CAD build for the part. Positions are in the model's coordinates, mm. A direction names the side the tool comes from. Coordinates: 2 decimals unless noted, no trailing zeros. Order: outer loops, then holes, each group sorted by start corner. A loop starts at its lowest first (then second) coordinate and runs counter-clockwise, first axis right, second up. Notation, with made-up numbers: (20.25, 67.5) - (29.25, 67.5) arc R24 cw to (29.25, 80.5) - close; hole circle Ø7 at (43, 60.25). An arc over 180 degrees is marked (long way). Return JSON: item names as keys, results as strings.
from build123d import *

# Parameters (mm, degrees)
SKETCH1_R           = 5
BOSS_EXTRUDE1_DEPTH = 6
SKETCH2_R           = 13
CUT_EXTRUDE1_DEPTH  = 3
CUT_EXTRUDE1_DRAFT  = -30
SKETCH3_R           = 18
BOSS_EXTRUDE2_DEPTH = 48
SKETCH4_R           = 38
BOSS_EXTRUDE3_DEPTH = 10
SKETCH5_R           = 11.267949192
CUT_EXTRUDE2_DEPTH  = 25
SKETCH6_R           = 10
CUT_EXTRUDE3_DEPTH  = 76.55130707
SKETCH7_R           = 4
CUT_EXTRUDE4_DEPTH  = 87.856203002
FILLET1_R           = 2


with BuildPart() as part:
    # Sketch1 → Boss-Extrude1 (new, symmetric)
    with BuildSketch(Plane.XY):
        with BuildLine():
            Line((23.491540883, -8.552631579), (11.275939624, -42.105263158))
            ThreePointArc((11.275939624, -42.105263158), (0, -50), (-11.275939624, -42.105263158))
            Line((-11.275939624, -42.105263158), (-23.491540883, -8.552631579))
            ThreePointArc((-23.491540883, -8.552631579), (-25, 0), (-23.491540883, 8.552631579))
            Line((-23.491540883, 8.552631579), (-11.275939624, 42.105263158))
            ThreePointArc((-11.275939624, 42.105263158), (0, 50), (11.275939624, 42.105263158))
            Line((11.275939624, 42.105263158), (23.491540883, 8.552631579))
            ThreePointArc((23.491540883, 8.552631579), (25, 0), (23.491540883, -8.552631579))
        make_face()
        with Locations((0, -38)):
            Circle(SKETCH1_R, mode=Mode.SUBTRACT)
        with Locations((0, 38)):
            Circle(SKETCH1_R, mode=Mode.SUBTRACT)
    extrude(amount=BOSS_EXTRUDE1_DEPTH, both=True)


with BuildPart() as cut_extrude1_tool:
    # Sketch2 → Cut-Extrude1 (with draft: the straight prism first)
    with BuildSketch(Plane.XY.offset(6)):
        Circle(SKETCH2_R)
    extrude(amount=-CUT_EXTRUDE1_DEPTH)
    # Cut-Extrude1: the draft: its side faces are tilted about the plane it starts from
    cut_extrude1_sides = [cut_extrude1_tool.faces().sort_by_distance(p)[0] for p in [
        (-13, 0, 4.5),
    ]]
    draft(cut_extrude1_sides, Plane.XY.offset(6), CUT_EXTRUDE1_DRAFT)


with BuildPart() as part_1:
    add(part.part)

    # Cut-Extrude1: cut by cut_extrude1_tool
    add(cut_extrude1_tool.part, mode=Mode.SUBTRACT)

    # Sketch3 → Boss-Extrude2 (add)
    with BuildSketch(Plane(origin=(0, 0, -6), x_dir=(-1, 0, 0), z_dir=(0, 0, -1))):
        with Locations(Location((0, 0, 0), (0, 0, 180))):
            Circle(SKETCH3_R)
    extrude(amount=BOSS_EXTRUDE2_DEPTH)

    # Sketch4 → Boss-Extrude3 (add)
    with BuildSketch(Plane(origin=(0, 0, -54), x_dir=(-1, 0, 0), z_dir=(0, 0, -1))):
        Circle(SKETCH4_R)
    extrude(amount=BOSS_EXTRUDE3_DEPTH)

    # Sketch5 → Cut-Extrude2 (cut)
    with BuildSketch(Plane.XY.offset(3)):
        Circle(SKETCH5_R)
    extrude(amount=-CUT_EXTRUDE2_DEPTH, mode=Mode.SUBTRACT)

    # Sketch6 → Cut-Extrude3 (cut, through all)
    with BuildSketch(Plane.XY.offset(-22)):
        Circle(SKETCH6_R)
    extrude(amount=-CUT_EXTRUDE3_DEPTH, mode=Mode.SUBTRACT)

    # Sketch7 → Cut-Extrude4 (cut, through all)
    with BuildSketch(Plane.XY.offset(-54)):
        with Locations((0, 29)):
            Circle(SKETCH7_R)
        with Locations((25.11473671, 14.5)):
            Circle(SKETCH7_R)
        with Locations((25.11473671, -14.5)):
            Circle(SKETCH7_R)
        with Locations((0, -29)):
            Circle(SKETCH7_R)
        with Locations((-25.11473671, -14.5)):
            Circle(SKETCH7_R)
        with Locations((-25.11473671, 14.5)):
            Circle(SKETCH7_R)
    extrude(amount=-CUT_EXTRUDE4_DEPTH, mode=Mode.SUBTRACT)

    # Fillet1
    fillet1_edges = [part_1.edges().sort_by_distance(p)[0] for p in [
        (-18, 0, -54),
        (38, 0, -54),
    ]]
    fillet(fillet1_edges, radius=FILLET1_R)


solid = part_1.part
Item 1: Drop flat-ended pins along their axis: P1, Ø6, axis at x = 16, z = -18.5, coming from the -Y side; P2, Ø12, axis at y = -3, z = -34.5, coming from the -X side; P3, Ø12, axis at x = -2, z = -31.5, coming from the +Y side. Give the stop position or say it passes through.
Findings below:
{"P1": "stops at y = -12.45", "P2": "stops at x = -18", "P3": "stops at y = 18"}
Item 2: Band-saw the part on C-C, the plane z = -48. List the corners of the cut face in (x, y), then the cut area to 3 significant figures.
Findings below:
{"outline": "circle Ø36 at (0, 0); hole circle Ø20 at (0, 0)", "area": "704 mm²"}
Item 3: Band-saw the part on A-A, the plane z = 0. List the corners of the cut face in (x, y), then the cut area to 3 significant figures.
Findings below:
{"outline": "(-23.49, -8.55) - (-11.28, -42.11) arc R12 ccw to (11.28, -42.11) - (23.49, -8.55) arc R25 ccw to (23.49, 8.55) - (11.28, 42.11) arc R12 ccw to (-11.28, 42.11) - (-23.49, 8.55) arc R25 ccw to start; hole circle Ø22.54 at (0, 0); hole circle Ø10 at (0, -38); hole circle Ø10 at (0, 38)", "area": "2,870 mm²"}
Item 4: Band-saw the part on B-B, the plane x = 0. Count the separate pieces of the cut face and the enclosed holes in it, then the cut area to 3 significant figures.
Findings below:
{"separate pieces": "6", "enclosed holes": "0", "area": "1,810 mm²"}
Item 5: Wall check: L1, parallel to Y at x = 0, z = -61.5; L2, parallel to X at y = 14, z = -58; L3, parallel to Z at x = 5.5, y = 38.5. Give the ranges that are in metal, low to high. Write a range as [from, to].
Findings below:
{"L1": "y = [-38, -33], [-25, -10], [10, 25], [33, 38]", "L2": "x = [-35.33, -29.08], [-21.15, 21.15], [29.08, 35.33]", "L3": "z = [-6, 6]"}
Item 6: Mould opens along X. For faces 4 (the cylindrical face through (28.81, -16.03, -58.93)), 5 (the cylindrical face through (-25, 0, 0)), 6 (the cylindrical face through (0, 50, 0)) say: released by +X, released by -X, zero draft, split by the parting line, or undercut.
Findings below:
{"face 4": "undercut", "face 5": "released by -X", "face 6": "split by the parting line"}
Item 7: Which spindle directions (+Z, -Z, +X, -X, +Y, -Y) get a long thin tool onto all of the face, cutting with end or side? Do faces 1 (the cylindrical face through (10.75, 3.38, -9.32)), 2 (the flat face through (17.3, 25.56, 0.08)), 3 (the flat face through (-17.3, -25.56, 0.08)). Say none if no direction does.
Findings below:
{"face 1": "+Z", "face 2": "+Z, +X, +Y", "face 3": "+Z, -X, -Y"}
